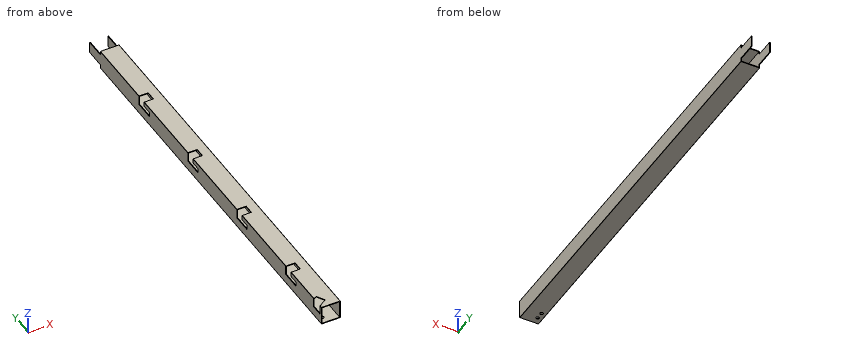
```python
from build123d import *

# Parameters (mm, degrees)
SKETCH1_W           = 37
SKETCH1_H           = 37
BOSS_EXTRUDE1_DEPTH = 899
CUT_EXTRUDE2_DEPTH  = 20
SKETCH4_W           = 8
SKETCH4_H           = 41
CUT_EXTRUDE3_DEPTH  = 901.777997067
SKETCH5_R           = 3.5
CUT_EXTRUDE4_DEPTH  = 10
CUT_EXTRUDE5_DEPTH  = 20


with BuildPart() as part:
    # Sketch1 → Boss-Extrude1 (new body)
    with BuildSketch(Plane(origin=(0, 0, 0), x_dir=(1, 0, 0), z_dir=(0, 1, 0))):
        with BuildLine():
            Line((0.5, 0), (39.5, 0))
            ThreePointArc((39.5, 0), (39.853553391, 0.146446609), (40, 0.5))
            Line((40, 0.5), (40, 39.5))
            ThreePointArc((40, 39.5), (39.853553391, 39.853553391), (39.5, 40))
            Line((39.5, 40), (0.5, 40))
            ThreePointArc((0.5, 40), (0.146446609, 39.853553391), (0, 39.5))
            Line((0, 39.5), (0, 0.5))
            ThreePointArc((0, 0.5), (0.146446609, 0.146446609), (0.5, 0))
        make_face()
        with Locations((20, 20)):
            Rectangle(SKETCH1_W, SKETCH1_H, mode=Mode.SUBTRACT)
    extrude(amount=BOSS_EXTRUDE1_DEPTH)

    # Sketch3 → Cut-Extrude2 (cut)
    with BuildSketch(Plane.XY):
        Polygon((0, 29.014346333), (0, 5.907288086), (3, 5.907288086), (3, 7.639845548), (17.125490967, 15.797587142), (7.072929751, 33.098592085), (3, 30.74639714), (0, 30.74639714), align=None)
    extrude(amount=-CUT_EXTRUDE2_DEPTH, mode=Mode.SUBTRACT)

    # Sketch4 → Cut-Extrude3 (cut, through all)
    with BuildSketch(Plane.ZY):
        with Locations((-4, 878.5)):
            Rectangle(SKETCH4_W, SKETCH4_H)
        with Locations((-36, 878.5)):
            Rectangle(SKETCH4_W, SKETCH4_H)
    extrude(amount=-CUT_EXTRUDE3_DEPTH, mode=Mode.SUBTRACT)

    # Sketch5 → Cut-Extrude4 (cut)
    with BuildSketch(Plane(origin=(0, 0, -40), x_dir=(-1, 0, 0), z_dir=(0, 0, -1))):
        with Locations((-10, 30)):
            Circle(SKETCH5_R)
        with Locations((-10, 15)):
            Circle(SKETCH5_R)
    extrude(amount=-CUT_EXTRUDE4_DEPTH, mode=Mode.SUBTRACT)

    # Sketch6 → Cut-Extrude5 (cut)
    with BuildSketch(Plane.ZY):
        Polygon((0, 708.5), (-20, 708.5), (-20, 668), (-10, 668), (-10, 688), (0, 688), align=None)
        Polygon((0, 518.5), (-20, 518.5), (-20, 478), (-10, 478), (-10, 498), (0, 498), align=None)
        Polygon((0, 328.5), (-20, 328.5), (-20, 288), (-10, 288), (-10, 308), (0, 308), align=None)
        Polygon((0, 138.5), (-20, 138.5), (-20, 98), (-10, 98), (-10, 118), (0, 118), align=None)
    extrude(amount=-CUT_EXTRUDE5_DEPTH, mode=Mode.SUBTRACT)


solid = part.part
```
Part model, mm, in its own coordinate system. Give positions to 0.01 mm unless a question says otherwise; leave off trailing zeros. Write each loop counter-clockwise with the first axis right and the second up, starting at its lowest first coordinate (ties: lowest second). Pieces come first, ordered by that corner, then holes. Notation, with made-up numbers: M -26.75,35 L 22.25,35 A22 cw 22.25,73 Z; hole C 61.25,27.25 d10. An arc over 180 degrees is marked long. Use CSV: the item, a comma, the result in double quotes.
Item 1: Slice it at A-A on y = 240.5. Write the cut outline in (x, z), plus the area to 3 significant figures.
Taken from the geometry:
outline,"M 0,-39.5 A0.5 ccw 0.5,-40 L 39.5,-40 A0.5 ccw 40,-39.5 L 40,-0.5 A0.5 ccw 39.5,0 L 0.5,0 A0.5 ccw 0,-0.5 Z; hole M 1.5,-38.5 L 38.5,-38.5 L 38.5,-1.5 L 1.5,-1.5 Z"
area,"231 mm²"
Item 2: Pin check, flat tips, straight feed: P1, Ø8, axis at x = 6, z = -3, coming from the +Y side; P2, Ø1.6, axis at y = 317.5, z = -1, coming from the -X side. Stop position of each tip, or through.
Taken from the geometry:
P1,"stops at y = 858"
P2,"stops at x = 20"
Item 3: Drill centre lines: probe 1 along Y at (x, z) = (10, -39); probe 2 along Z at (x, y) = (31.5, 55); probe 3 along X at (y, z) = (68.5, -18). Where is each one in solid material? Low to high.
Taken from the geometry:
probe 1,"y = 0 to 11.5, 18.5 to 26.5, 33.5 to 858"
probe 2,"z = -40 to -38.5, -1.5 to 0"
probe 3,"x = 0 to 1.5, 38.5 to 40"
Item 4: Slice it at B-B on x = 27.5. Write the cut outline in (y, z), plus the area to 3 significant figures.
Taken from the geometry:
outline,"M 0,-40 L 858,-40 L 858,-38.5 L 0,-38.5 Z; M 0,-1.5 L 858,-1.5 L 858,0 L 0,0 Z"
area,"2,570 mm²"
